Read the model definition and answer for the solid it produces. Units are mm, in the model's axes. A direction names the side the tool comes from. Coordinates: 2 decimals unless noted, no trailing zeros. Order: outer loops, then holes, each group sorted by start corner. A loop starts at its lowest first (then second) coordinate and runs counter-clockwise, first axis right, second up. Notation, with made-up numbers: (-13.75, -23) -> (27.25, -23) arc R20 cw to (27.25, -5) -> close; hole circle Ø1 at (5, 39). An arc over 180 degrees is marked (long way). Return JSON: item names as keys, results as strings. Group by question number.
```python
from build123d import *

# Parameters (mm, degrees)
SKETCH039_R     = 1
PAD010_DEPTH    = 1.35
SKETCH041_W     = 2
SKETCH041_H     = 1
PAD014_DEPTH    = 4.35
SKETCH040_W     = 2.7
SKETCH040_H     = 3
PAD015_DEPTH    = 0.85
POCKET015_DEPTH = 5.351
FILLET_R        = 0.1


with BuildPart() as part:
    # Sketch039 → Pad010 (new body)
    with BuildSketch(Plane.YZ.offset(-1.5)):
        with BuildLine():
            ThreePointArc((4.2, 7), (0, 11.2), (-4.2, 7))
            Line((-4.2, 7), (-4.2, 0.5))
            Line((-4.2, 0.5), (4.2, 0.5))
            Line((4.2, 0.5), (4.2, 7))
        make_face()
        with Locations((0, 7)):
            Circle(SKETCH039_R, mode=Mode.SUBTRACT)
    extrude(amount=PAD010_DEPTH)

    # Sketch041 → Pad014 (join)
    with BuildSketch(Plane.YZ.offset(-1.5)):
        with Locations((0, 1)):
            Rectangle(SKETCH041_W, SKETCH041_H)
    extrude(amount=-PAD014_DEPTH)

    # Sketch040 (on Face7 of Pad010) → Pad015 (join)
    with BuildSketch(Plane.YZ.offset(-0.15)):
        with Locations((-2.85, 2)):
            Rectangle(SKETCH040_W, SKETCH040_H)
        with Locations((2.85, 2)):
            Rectangle(SKETCH040_W, SKETCH040_H)
    extrude(amount=PAD015_DEPTH)

    # Sketch055 → Pocket015 (cut, through all)
    with BuildSketch(Plane.YZ.offset(-0.5)):
        Polygon((-2.5, 4.7), (4, 4.7), (4, 4.4), (2.5, 4.4), (2.5, 1.8), (-2.5, 1.8), align=None)
    extrude(amount=-POCKET015_DEPTH, mode=Mode.SUBTRACT)

    # Fillet
    fillet_edges = [part.edges().sort_by_distance(p)[0] for p in [
        (0.275, -4.2, 3.5),
        (0.7, -2.85, 3.5),
        (0.7, -1.5, 2),
        (0.7, -2.85, 0.5),
        (0.7, -4.2, 2),
        (0.7, 2.85, 3.5),
        (0.7, 4.2, 2),
        (0.7, 2.85, 0.5),
        (0.7, 1.5, 2),
    ]]
    fillet(fillet_edges, radius=FILLET_R)


with BuildPart() as part_1:
    # Body010 placement: moved
    add(part.part.moved(Location((0, 0, -0.5))))


solid = part_1.part
```
1. Straight lines are drawn through the part: L1, parallel to Z at x = -0.6, y = 0; L2, parallel to X at y = -3.25, z = 2.5; L3, parallel to Z at x = 0, y = 2.5. For each, find the intervals that lie inside material, in ascending order.
2. Given pin 1 (1.1 mm diameter, centred on x = -3, z = 0.5, fed in from -Y); pin 2 (1.1 mm diameter, centred on x = -1, y = 3, fed in from +Z); pin 3 (0.8 mm diameter, centred on x = 0.5, y = -2.5, fed in from +Z); pin 4 (1 mm diameter, centred on x = -5, y = -2.5, fed in from +Z), each flat-ended and moving along its own axis, determine where each tip first touches the part or whether it passes through.
3. Find section B-B on z = 6.25. Determine the outline of the cut face in (x, y).
4. Find section A-A on y = 0. Determine the outline of the cut face in (x, z), and give its area (3 significant figures).
5. Which of the six approach directions +Z, -Z, +X, -X, +Y, -Y give full straight-line access (tool end or side, diameter ignored) to faces 1 (the face through (-3.6, 1, 0.5)), 2 (the face through (-1, 3, 3.9)), 3 (the face through (-3.6, -1, 0.5))?
6. For a pull along Z with two mould halves and no side action, classify faces 4 (the face through (-2, 0, 0)), 5 (the face through (-1, 0, 1.3)), 6 (the face through (-0.15, 0, 5)) as released by +Z, released by -Z, zero draft, split by the parting line, or undercut.
7. Find section C-C on x = -1. Determine the outline of the cut face in (y, z).
8. Find section D-D on y = 2. Determine the outline of the cut face in (x, z), and give its area (3 significant figures).
Result:
{
 "1": {"L1": "0 to 1.3, 4.2 to 5.5, 7.5 to 10.7", "L2": "-1.5 to 0.7", "L3": "0 to 3"},
 "2": {"pin 1": "y = -1", "pin 2": "z = 9.91", "pin 3": "z = 3", "pin 4": "through"},
 "3": {"outline": "(-1.5, -4.2) -> (-0.15, -4.2) -> (-0.15, -0.97) -> (-1.5, -0.97) -> close; (-1.5, 0.97) -> (-0.15, 0.97) -> (-0.15, 4.2) -> (-1.5, 4.2) -> close"},
 "4": {"outline": "(-5.85, 0) -> (-0.15, 0) -> (-0.15, 5.5) -> (-1.5, 5.5) -> (-1.5, 4.2) -> (-0.5, 4.2) -> (-0.5, 1.3) -> (-1.5, 1.3) -> (-1.5, 1) -> (-5.85, 1) -> close; (-1.5, 7.5) -> (-0.15, 7.5) -> (-0.15, 10.7) -> (-1.5, 10.7) -> close", "area": "13.2 mm^2"},
 "5": {"face 1": "+Z, -Z, -X, +Y", "face 2": "-X", "face 3": "+Z, -Z, -X, -Y"},
 "6": {"face 4": "released by -Z", "face 5": "undercut", "face 6": "zero draft"},
 "7": {"outline": "(-4.2, 0) -> (4.2, 0) -> (4.2, 6.5) arc R4.2 ccw to (-4.2, 6.5) -> close; hole (-2.5, 1.3) -> (2.5, 1.3) -> (2.5, 3.9) -> (4, 3.9) -> (4, 4.2) -> (-2.5, 4.2) -> close; hole circle Ø2 at (0, 6.5)"},
 "8": {"outline": "(-1.5, 0) -> (0.6, 0) arc R0.1 ccw to (0.7, 0.1) -> (0.7, 2.9) arc R0.1 ccw to (0.6, 3) -> (-0.15, 3) -> (-0.15, 10.19) -> (-1.5, 10.19) -> (-1.5, 4.2) -> (-0.5, 4.2) -> (-0.5, 1.3) -> (-1.5, 1.3) -> close", "area": "13.4 mm^2"}
}
